Read the model definition and answer for the solid it produces. Units are mm, in the model's axes. A direction names the side the tool comes from. Round coordinates to 2 decimals unless told otherwise and drop trailing zeros. Write each loop counter-clockwise with the first axis right and the second up, starting at its lowest first coordinate (ties: lowest second). Pieces come first, ordered by that corner, then holes. Notation, with made-up numbers: (-1, 5) -> (14, 5) arc R22 cw to (14, 44) -> close; hole circle Ø4 at (69, -24.75). An arc over 180 degrees is marked (long way). Return JSON: item names as keys, results as strings. Group by question number.
(1) A cutting plane is placed at B-B on x = -71. Give the vertices of the cut face in (y, z).
(2) A cutting plane is placed at D-D on z = 15.5. Give the vertices of the cut face in (x, y), then the cut area to 3 significant figures.
(3) The mould has two halves that part along X. Classify faces 4 (the flat face through (124, -51, 0)), 5 (the flat face through (0, 0, 44.45)): released by +X, released by -X, zero draft, split by the parting line, or undercut.
(4) Given pin 1 (1.9 mm diameter, centred on x = -25.5, y = -26, fed in from +Z); pin 2 (6 mm diameter, centred on y = 85, z = 36, fed in from -X); pin 3 (10 mm diameter, centred on x = -8.98, y = -8.98, fed in from -Z); pin 4 (5 mm diameter, centred on x = 40.5, z = 35, fed in from -Y), each flat-ended and moving along its own axis, determine where each tip first touches the part or whether it passes through.
(5) A cutting plane is placed at A-A on z = 39. Give the vertices of the cut face in (x, y) (3 decimals), then the cut area to 3 significant figures.
(6) A cutting plane is placed at C-C on y = 71. Give the vertices of the cut face in (x, z).
(7) For faces 1 (the flat face through (-19, -19, 30.956)), 2 (the cylindrical face through (-47.26, 48.9, 38.19)), 3 (the flat face through (0, 38, 44.45)), determine the directions among +Z, -Z, +X, -X, +Y, -Y from which every point of the face is accessible in a straight line to the end or side of a thin tool.
(8) Straight lines are drawn through the part: line 1 (X direction, y = -2, z = 70); line 2 (X direction, y = 35.5, z = 40); line 3 (Y direction, x = -53.5, z = 44). For each, find the intervals that lie inside material, in ascending order.
Autodesk Inventor part; units mm, degrees
ref_plane "Work Plane1" through (0, 0, 38.1) normal (0, 0, 1) x (1, 0, 0)
ref_plane "Work Plane2" through (0, 0, 44.45) normal (0, 0, 1) x (1, 0, 0)
ref_plane "YZ Plane" through (0, 0, 0) normal (1, 0, 0) x (0, 1, 0)
sketch "Sketch1" plane through (0, 0, 0) normal (0, 0, 1) x (1, 0, 0)
  circle A0 centre (0, 0) radius 139.7
  circle A1 centre (0, 0) radius 133.35
  dimension "d0" = 279.4
  dimension "d1" = 266.7
extrude "Extrusion1" add sketch "Sketch1" along normal blind 76.2
ref_plane "Work Plane1" through (0, 0, 38.1) normal (0, 0, 1) x (1, 0, 0)
sketch "Sketch2" plane through (0, 0, 38.1) normal (0, 0, 1) x (1, 0, 0)
  circle A0 centre (0, 0) radius 133.35
  circle A1 centre (0, 0) radius 120.65
  dimension "d5" = 241.3
extrude "Extrusion2" add sketch "Sketch2" along normal mid plane 79.375
ref_plane "Work Plane2" through (0, 0, 44.45) normal (0, 0, 1) x (1, 0, 0)
sketch "Sketch3" plane through (0, 0, 44.45) normal (0, 0, 1) x (1, 0, 0)
  circle A0 centre (0, 0) radius 120.65
  circle A1 centre (0, 82.55) radius 25.4
  line L0 (0, 82.55) -> (0, 0) construction
  circle A2 centre (-71.4904, 41.275) radius 25.4
  line L1 (-71.4904, 41.275) -> (0, 0) construction
  circle A3 centre (-71.4904, -41.275) radius 25.4
  line L2 (-71.4904, -41.275) -> (0, 0) construction
  circle A4 centre (0, -82.55) radius 25.4
  line L3 (0, -82.55) -> (0, 0) construction
  circle A5 centre (71.4904, -41.275) radius 25.4
  line L4 (71.4904, -41.275) -> (0, 0) construction
  circle A6 centre (71.4904, 41.275) radius 25.4
  line L5 (71.4904, 41.275) -> (0, 0) construction
  dimension "d11" = 241.3
  dimension "d12" = 50.8
  dimension "d13" = 82.55
  dimension "d16" = 360
extrude "Extrusion3" add sketch "Sketch3" against normal blind 12.7
sketch "Sketch4" plane through (0, 0, 44.45) normal (0, 0, 1) x (1, 0, 0)
  circle A0 centre (0, 0) radius 44.45
  dimension "d20" = 88.9
extrude "Extrusion4" add sketch "Sketch4" along normal blind 8.4667
sketch "Sketch6" plane through (0, 0, 31.75) normal (0, 0, -1) x (-1, 0, 0)
  circle A0 centre (0, 0) radius 44.45
extrude "Extrusion5" add sketch "Sketch6" along normal blind 0.7937
sketch "Sketch5" plane through (0, 0, 52.9167) normal (0, 0, 1) x (1, 0, 0)
  circle A0 centre (-38.1, 0) radius 3.175
  circle A1 centre (38.1, 0) radius 3.175
  circle A2 centre (0, 38.1) radius 3.175
  circle A3 centre (0, -38.1) radius 3.175
  circle A4 centre (-26.9408, 26.9408) radius 3.175
  circle A5 centre (26.9408, 26.9408) radius 3.175
  circle A6 centre (26.9408, -26.9408) radius 3.175
  circle A7 centre (-26.9408, -26.9408) radius 3.175
  line L0 (-38.1, 0) -> (0, 0) construction
  line L1 (0, 0) -> (-26.9408, 26.9408) construction
  line L2 (0, 38.1) -> (0, 0) construction
  line L3 (26.9408, 26.9408) -> (0, 0) construction
  line L4 (38.1, 0) -> (0, 0) construction
  line L5 (26.9408, -26.9408) -> (0, 0) construction
  line L6 (0, -38.1) -> (0, 0) construction
  line L7 (-26.9408, -26.9408) -> (0, 0) construction
  line L8 (-8.9803, 8.9803) -> (8.9803, 8.9803) construction
  line L9 (8.9803, 8.9803) -> (8.9803, -8.9803) construction
  line L10 (8.9803, -8.9803) -> (-8.9803, -8.9803) construction
  line L11 (-8.9803, -8.9803) -> (-8.9803, 8.9803) construction
  circle A8 centre (-8.9803, 8.9803) radius 6.35
  circle A9 centre (8.9803, 8.9803) radius 6.35
  circle A10 centre (8.9803, -8.9803) radius 6.35
  circle A11 centre (-8.9803, -8.9803) radius 6.35
  dimension "d23" = 45
  dimension "d24" = 6.35
  dimension "d25" = 38.1
  dimension "d26" = 12.7
  dimension "d27" = 12.7
extrude "Extrusion6" cut sketch "Sketch5" against normal blind 8.4667
sketch "Sketch7" plane through (0, 0, 30.9563) normal (0, 0, -1) x (-1, 0, 0)
  circle A0 centre (0, 0) radius 25.4
  dimension "d32" = 50.8
extrude "Extrusion7" cut sketch "Sketch7" against normal blind 13.4938
properties part number "Main Wheel"
Checks:
{
 "1": {"outline": "(-120.31, 0) -> (-112.88, 0) -> (-112.88, -1.59) -> (-97.55, -1.59) -> (-97.55, 31.75) -> (-66.67, 31.75) -> (-66.67, 44.45) -> (-97.55, 44.45) -> (-97.55, 77.79) -> (-112.88, 77.79) -> (-112.88, 76.2) -> (-120.31, 76.2) -> close; (-15.88, 31.75) -> (15.88, 31.75) -> (15.88, 44.45) -> (-15.88, 44.45) -> close; (66.67, 31.75) -> (97.55, 31.75) -> (97.55, -1.59) -> (112.88, -1.59) -> (112.88, 0) -> (120.31, 0) -> (120.31, 76.2) -> (112.88, 76.2) -> (112.88, 77.79) -> (97.55, 77.79) -> (97.55, 44.45) -> (66.67, 44.45) -> close"},
 "2": {"outline": "circle Ø279.4 at (0, 0); hole circle Ø241.3 at (0, 0)", "area": "15,600 mm^2"},
 "3": {"face 4": "zero draft", "face 5": "undercut"},
 "4": {"pin 1": "stops at z = 44.45", "pin 2": "stops at x = -113.1", "pin 3": "passes through", "pin 4": "stops at y = -134.43"},
 "5": {"outline": "circle Ø279.4 at (0, 0); hole circle Ø50.8 at (-71.49, -41.275); hole circle Ø50.8 at (-71.49, 41.275); hole circle Ø50.8 at (0, -82.55); hole circle Ø50.8 at (0, 0); hole circle Ø50.8 at (0, 82.55); hole circle Ø50.8 at (71.49, -41.275); hole circle Ø50.8 at (71.49, 41.275)", "area": "47,100 mm^2"},
 "6": {"outline": "(-120.31, 0) -> (-112.88, 0) -> (-112.88, -1.59) -> (-97.55, -1.59) -> (-97.55, 31.75) -> (-22.62, 31.75) -> (-22.62, 44.45) -> (-97.55, 44.45) -> (-97.55, 77.79) -> (-112.88, 77.79) -> (-112.88, 76.2) -> (-120.31, 76.2) -> close; (22.62, 31.75) -> (97.55, 31.75) -> (97.55, -1.59) -> (112.88, -1.59) -> (112.88, 0) -> (120.31, 0) -> (120.31, 76.2) -> (112.88, 76.2) -> (112.88, 77.79) -> (97.55, 77.79) -> (97.55, 44.45) -> (22.62, 44.45) -> close"},
 "7": {"face 1": "-Z", "face 2": "+Z, -Z", "face 3": "+Z"},
 "8": {"line 1": "x = -139.69 to -120.63, 120.63 to 139.69", "line 2": "x = -135.11 to -96.23, -46.76 to 46.76, 96.23 to 135.11", "line 3": "y = -129.05 to -59.21, -23.34 to 23.34, 59.21 to 129.05"}
}
